```python
from build123d import *

# Parameters (mm, degrees)
BOSS_EXTRUDE1_DEPTH = 61.9125
FILLET1_R           = 0.762


with BuildPart() as part:
    # Sketch1 → Boss-Extrude1 (new body, symmetric)
    with BuildSketch(Plane(origin=(0, 0, 0), x_dir=(0, 0, -1), z_dir=(1, 0, 0))):
        Polygon((-1.3208, 0), (1.3208, 0), (1.3208, -2.8448), (1.143, -2.8448), (2.38125, -22.6568), (-2.38125, -22.6568), (-1.143, -2.8448), (-1.3208, -2.8448), align=None)
    extrude(amount=BOSS_EXTRUDE1_DEPTH, both=True)

    # Fillet1
    fillet1_edges = [part.edges().sort_by_distance(p)[0] for p in [
        (0, 0, 1.3208),
        (0, 0, -1.3208),
    ]]
    fillet(fillet1_edges, radius=FILLET1_R)


solid = part.part
```
Model file for the job. Use its own axes, mm. A direction names the side the tool comes from. Give positions to 0.01 mm unless a question says otherwise; leave off trailing zeros. Write each loop counter-clockwise with the first axis right and the second up, starting at its lowest first coordinate (ties: lowest second). Pieces come first, ordered by that corner, then holes. Notation, with made-up numbers: (86.25, 86) - (141.25, 86) arc R31 ccw to (141.25, 123) - close; hole circle Ø8 at (6, 36). An arc over 180 degrees is marked (long way). One line per question, with ' | ' between items. Start each with the question number.
(1) Wall check: line 1 along Z through (x, y) = (-3, -3); line 2 along Z through (x, y) = (26.5, -1.75); line 3 along Y through (x, z) = (40.5, -0.9). Give the ranges that are in metal, low to high. Write a range as from..to.
(2) Pin check, flat tips, straight feed: P1, Ø8, axis at x = 45.5, y = -16.5, coming from the +Z side; P2, Ø2.5, axis at x = 27.5, y = -2, coming from the -Z side; P3, Ø0.6, axis at x = -3.5, y = -2, coming from the +Z side. Stop position of each tip, or through.
(3) Slice it at C-C on y = -6. Write the cut outline in (x, z).
(4) 3-axis set-ups, long thin cutter, end or side, ignore diameter. For faces 1 (the face through (1, -2, 1.321)), 2 (the face through (1, -2, -1.321)), 3 (the face through (61.912, -14, 0)): which of +Z, -Z, +X, -X, +Y, -Y reach the whole face in a straight line?
(5) Slice it at B-B on y = -20. Write the cut outline in (x, z).
(6) Slice it at A-A on x = -9. Write the cut outline in (y, z).
Results below:
1) line 1: -1.15..1.15 | line 2: -1.32..1.32 | line 3: -22.66..-0.08
2) P1: z = 2.25 | P2: z = -1.32 | P3: z = 1.32
3) outline: (-61.91, -1.34) - (61.91, -1.34) - (61.91, 1.34) - (-61.91, 1.34) - close
4) face 1: +Z, +X, -X, +Y | face 2: -Z, +X, -X, +Y | face 3: +Z, -Z, +X, +Y, -Y
5) outline: (-61.91, -2.22) - (61.91, -2.22) - (61.91, 2.22) - (-61.91, 2.22) - close
6) outline: (-22.66, -2.38) - (-2.84, -1.14) - (-2.84, -1.32) - (-0.76, -1.32) arc R0.76 ccw to (0, -0.56) - (0, 0.56) arc R0.76 ccw to (-0.76, 1.32) - (-2.84, 1.32) - (-2.84, 1.14) - (-22.66, 2.38) - close
